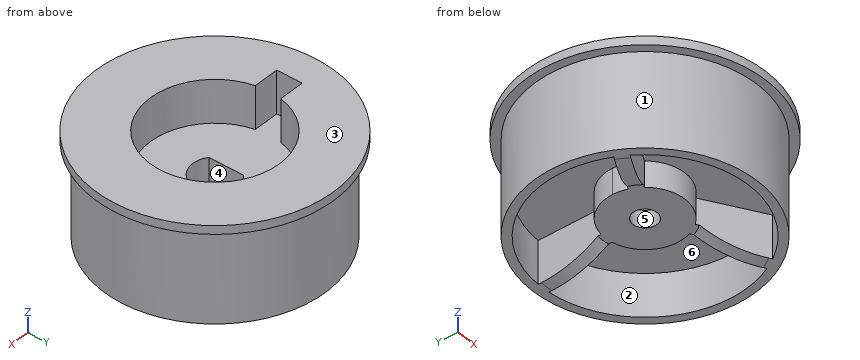
```python
from build123d import *

# Parameters (mm, degrees)
SKETCH_1_R          = 13
SKETCH_1_R_2        = 2.6
SKETCH_1_R_3        = 1.4
EXTRUDE_1_DEPTH     = 4
SKETCH_1_3_R        = 13
SKETCH_1_3_R_2      = 2.6
EXTRUDE_2_DEPTH     = 12
EXTRUDE_START       = 11
SKETCH_1_6_R        = 14
SKETCH_1_6_R_2      = 13
EXTRUDE_3_DEPTH     = 1
CUT_EXTRUDE_1_DEPTH = 5
SKETCH_6_R          = 7.6
SKETCH_6_W          = 3
SKETCH_6_H          = 3
CUT_EXTRUDE_5_DEPTH = 5
SKETCH_5_R          = 5
CUT_EXTRUDE_6_DEPTH = 2
FILLET_1_R          = 12


with BuildPart() as part:
    # 草图1 → 凸台-拉伸1 (new body)
    # profile 1 of 3: a face of its own
    with BuildSketch(Plane.XY):
        Circle(SKETCH_1_R)
        Circle(SKETCH_1_R_2, mode=Mode.SUBTRACT)
    # profile 2 of 3: a face of its own
    with BuildSketch(Plane.XY):
        with BuildLine():
            Line((-1.6, -2.049390153), (-1.6, 2.049390153))
            ThreePointArc((-1.6, 2.049390153), (-2.6, 0), (-1.6, -2.049390153))
        make_face()
    # profile 3 of 3: a face of its own
    with BuildSketch(Plane.XY):
        with BuildLine():
            ThreePointArc((2.6, 0), (1.140175425, 2.336664289), (-1.6, 2.049390153))
            Line((-1.6, 2.049390153), (-1.6, -2.049390153))
            ThreePointArc((-1.6, -2.049390153), (1.140175425, -2.336664289), (2.6, 0))
        make_face()
        Circle(SKETCH_1_R_3, mode=Mode.SUBTRACT)
    extrude(amount=EXTRUDE_1_DEPTH)

    # 草图1<3> → 凸台-拉伸2 (add)
    # profile 1 of 2: a face of its own
    with BuildSketch(Plane.XY):
        Circle(SKETCH_1_3_R)
        Circle(SKETCH_1_3_R_2, mode=Mode.SUBTRACT)
    # profile 2 of 2: a face of its own
    with BuildSketch(Plane.XY):
        with BuildLine():
            Line((-1.6, -2.049390153), (-1.6, 2.049390153))
            ThreePointArc((-1.6, 2.049390153), (-2.6, 0), (-1.6, -2.049390153))
        make_face()
    extrude(amount=EXTRUDE_2_DEPTH)

    # 草图1<6> → 凸台-拉伸3 (add)
    with BuildSketch(Plane.XY.offset(EXTRUDE_START)):
        Circle(SKETCH_1_6_R)
        Circle(SKETCH_1_6_R_2, mode=Mode.SUBTRACT)
    extrude(amount=EXTRUDE_3_DEPTH)

    # 草图3 → 切除-拉伸1 (cut)
    with BuildSketch(Plane(origin=(0, 0, 0), x_dir=(-1, 0, 0), z_dir=(0, 0, -1))):
        with BuildLine():
            Line((-10.746987514, -5.338750731), (-4.305410284, -1.619704383))
            ThreePointArc((-4.305410284, -1.619704383), (-3.983716857, 2.3), (-0.75, 4.538446871))
            Line((-0.75, 4.538446871), (-0.75, 11.976539567))
            ThreePointArc((-0.75, 11.976539567), (-10.392304845, 6), (-10.746987514, -5.338750731))
        make_face()
        with BuildLine():
            Line((9.996987514, -6.637788836), (3.555410284, -2.918742488))
            ThreePointArc((3.555410284, -2.918742488), (0, -4.6), (-3.555410284, -2.918742488))
            Line((-3.555410284, -2.918742488), (-9.996987514, -6.637788836))
            ThreePointArc((-9.996987514, -6.637788836), (0, -12), (9.996987514, -6.637788836))
        make_face()
        with BuildLine():
            ThreePointArc((4.6, 0), (4.52575338, -0.823138109), (4.305410284, -1.619704383))
            Line((4.305410284, -1.619704383), (10.746987514, -5.338750731))
            ThreePointArc((10.746987514, -5.338750731), (11.682547885, -2.741910814), (12, 0))
            ThreePointArc((12, 0), (8.746427842, 8.215838363), (0.75, 11.976539567))
            Line((0.75, 11.976539567), (0.75, 4.538446871))
            ThreePointArc((0.75, 4.538446871), (3.507848343, 2.975735203), (4.6, 0))
        make_face()
    extrude(amount=-CUT_EXTRUDE_1_DEPTH, mode=Mode.SUBTRACT)

    # 草图6 → 切除-拉伸5 (cut)
    with BuildSketch(Plane.XY.offset(12)):
        Circle(SKETCH_6_R)
        with Locations((-8.950503339, 0)):
            Rectangle(SKETCH_6_W, SKETCH_6_H)
    extrude(amount=-CUT_EXTRUDE_5_DEPTH, mode=Mode.SUBTRACT)

    # 草图5 → 切除-拉伸6 (cut)
    with BuildSketch(Plane(origin=(0, 0, 0), x_dir=(-1, 0, 0), z_dir=(0, 0, -1))):
        Circle(SKETCH_5_R)
    extrude(amount=-CUT_EXTRUDE_6_DEPTH, mode=Mode.SUBTRACT)

    # 圆角1
    # the kernel refuses this fillet: 12 mm, written as the material it takes off along each edge
    with BuildSketch(Plane(origin=(0, 0, 0), x_dir=(-0.0031415874858860904, -0.9999950652018581, 0), z_dir=(0.9999950652018581, -0.0031415874858860904, 0))) as fillet_1_piece_1:
        with BuildLine():
            CenterArc((11.633249581, -12), FILLET_1_R, 90, 33.557309762)
            Line((5, -2), (5, 0))
            Line((5, 0), (11.633249581, 0))
        make_face()
    revolve(axis=Axis((0, 0, 0), (0, 0, -1)), revolution_arc=359.64, mode=Mode.SUBTRACT)
    with BuildSketch(Plane(origin=(0, 0, 0), x_dir=(0.8675919238668026, 0.49727683802998507, 0), z_dir=(-0.49727683802998507, 0.8675919238668026, 0))) as fillet_1_piece_2:
        with BuildLine():
            CenterArc((11.633249581, -12), FILLET_1_R, 90, 33.557309762)
            Line((5, -2), (5, 0))
            Line((5, 0), (11.633249581, 0))
        make_face()
    revolve(axis=Axis((0, 0, 0), (0, 0, -1)), revolution_arc=359.64, mode=Mode.SUBTRACT)
    with BuildSketch(Plane(origin=(0, 0, 0), x_dir=(-0.8644503363809427, 0.5027182271719167, 0), z_dir=(-0.5027182271719167, -0.8644503363809427, 0))) as fillet_1_piece_3:
        with BuildLine():
            CenterArc((11.633249581, -12), FILLET_1_R, 90, 33.557309762)
            Line((5, -2), (5, 0))
            Line((5, 0), (11.633249581, 0))
        make_face()
    revolve(axis=Axis((0, 0, 0), (0, 0, -1)), revolution_arc=359.64, mode=Mode.SUBTRACT)


solid = part.part
```
Build history of the part. All positions in model axes, mm. Face numbers are marked on the shaded views. A direction names the side the tool comes from. Give positions to 0.01 mm unless a question says otherwise; leave off trailing zeros. Loops run counter-clockwise (first coordinate to the right, second up) from the corner with the lowest first, then second, coordinate; pieces in that order, holes last. Notation, with made-up numbers: (65, -35) -> (88, -35) arc R27 ccw to (88, 0) -> close; hole circle Ø7 at (-25.75, 65.25). An arc over 180 degrees is marked (long way). One line per question, with ' | ' between items. Start each with the question number.
1) Cut at A-A (z = 6.5). Give the cut face in (x, y), plus the area to 3 significant figures.
2) Two-plate mould, pull along X, no slides. Class the marked faces 1, 2 and 3: released by +X, released by -X, zero draft, split by the parting line, or undercut.
3) Cut at B-B (y = 1). Give the cut face in (x, z), plus the area to 3 significant figures.
4) Cut at C-C (z = 10.5). Give the cut face in (x, y).
5) 3-axis set-ups, long thin cutter, end or side, ignore diameter. For the marked faces 4, 5 and 6: which of +Z, -Z, +X, -X, +Y, -Y reach the whole face in a straight line?
6) Pin check, flat tips, straight feed: pin 1 (1 mm diameter, centred on y = -3, z = 3, fed in from +X); pin 2 (1.5 mm diameter, centred on y = -0.5, z = 6, fed in from +X); pin 3 (3.5 mm diameter, centred on x = 0, y = -1, fed in from +Z). Stop position of each tip, or through.
7) Probe L1, parallel to Y at x = 0, z = 5.35; L2, parallel to X at y = -3.5, z = 2.5; L3, parallel to Y at x = 6.25, z = 3. List the from-to ranges inside material, lowest first.
Return value:
1) outline: circle Ø26 at (0, 0); hole (-1.6, -2.05) arc R2.6 ccw (long way) to (-1.6, 2.05) -> close | area: 513 mm^2
2) face 1: split by the parting line | face 2: undercut | face 3: zero draft
3) outline: (-13.96, 11) -> (-12.96, 11) -> (-12.96, 0) -> (-11.96, 0) -> (-11.96, 5) -> (-4.49, 5) -> (-4.49, 2) -> (-0.98, 2) -> (-0.98, 4) -> (-1.6, 4) -> (-1.6, 7) -> (-10.45, 7) -> (-10.45, 12) -> (-13.96, 12) -> close; (0.98, 2) -> (4.49, 2) -> (4.49, 5) -> (11.96, 5) -> (11.96, 0) -> (12.96, 0) -> (12.96, 11) -> (13.96, 11) -> (13.96, 12) -> (7.53, 12) -> (7.53, 7) -> (2.4, 7) -> (2.4, 4) -> (0.98, 4) -> close | area: 115 mm^2
4) outline: circle Ø26 at (0, 0); hole (-10.45, -1.5) -> (-7.45, -1.5) arc R7.6 ccw (long way) to (-7.45, 1.5) -> (-10.45, 1.5) -> close
5) face 4: +Z | face 5: +Z, -Z | face 6: -Z
6) pin 1: x = 12.76 | pin 2: x = 13 | pin 3: z = 7
7) L1: -13 to -2.6, 2.6 to 13 | L2: -12.52 to -11.48, -7.56 to -4.56, -2.98 to 2.98, 4.56 to 7.56, 11.48 to 12.52 | L3: -11.4 to -10.24, -4.47 to -2.74, 10.24 to 11.4
